Geometry check sheet. Reference: the model listing, model coordinates, mm. A direction names the side the tool comes from. Round coordinates to 2 decimals unless told otherwise and drop trailing zeros. Loops run counter-clockwise (first coordinate to the right, second up) from the corner with the lowest first, then second, coordinate; pieces in that order, holes last.
```python
from build123d import *

# Parameters (mm, degrees)
SKETCH_1_W          = 27.7
SKETCH_1_H          = 27.5
EXTRUDE_1_DEPTH     = 2
SKETCH_1_13_W       = 2
SKETCH_1_13_H       = 27.5
EXTRUDE_2_DEPTH     = 5
SKETCH_2_R          = 0.75
SKETCH_2_W          = 18
SKETCH_2_H          = 4.15
CUT_EXTRUDE_1_DEPTH = 22.196344024
SKETCH_2_3_W        = 25
SKETCH_2_3_H        = 19
CUT_EXTRUDE_2_DEPTH = 1
EXTRUDE_START       = 5
SKETCH_1_14_W       = 3
SKETCH_1_14_H       = 3
SKETCH_1_14_R       = 0.6
EXTRUDE_3_DEPTH     = 1.5


with BuildPart() as part:
    # 草图1 → 凸台-拉伸1 (new body)
    with BuildSketch(Plane.XY):
        Rectangle(SKETCH_1_W, SKETCH_1_H)
    extrude(amount=EXTRUDE_1_DEPTH)

    # 草图1<13> → 凸台-拉伸2 (add)
    with BuildSketch(Plane.XY):
        with Locations((-14.85, 0)):
            Rectangle(SKETCH_1_13_W, SKETCH_1_13_H)
        with Locations((14.85, 0)):
            Rectangle(SKETCH_1_13_W, SKETCH_1_13_H)
    extrude(amount=EXTRUDE_2_DEPTH)

    # 草图2 → 切除-拉伸1 (cut, through all)
    with BuildSketch(Plane.XY.offset(2)):
        with Locations((-11.7, 11.675)):
            Circle(SKETCH_2_R)
        with Locations((11.7, 11.675)):
            Circle(SKETCH_2_R)
        with Locations((-11.7, -11.675)):
            Circle(SKETCH_2_R)
        with Locations((11.7, -11.675)):
            Circle(SKETCH_2_R)
        with Locations((0, 11.675)):
            Rectangle(SKETCH_2_W, SKETCH_2_H)
    extrude(amount=-CUT_EXTRUDE_1_DEPTH, mode=Mode.SUBTRACT)

    # 草图2<3> → 切除-拉伸2 (cut)
    with BuildSketch(Plane.XY.offset(2)):
        with Locations((0, 0.1)):
            Rectangle(SKETCH_2_3_W, SKETCH_2_3_H)
    extrude(amount=-CUT_EXTRUDE_2_DEPTH, mode=Mode.SUBTRACT)

    # 草图1<14> → 凸台-拉伸3 (add)
    # profile 1 of 4: a face of its own
    with BuildSketch(Plane.XY.offset(EXTRUDE_START)):
        with Locations((-17.35, 12.25)):
            Rectangle(SKETCH_1_14_W, SKETCH_1_14_H)
        with Locations((-17.35, 12.25)):
            Circle(SKETCH_1_14_R, mode=Mode.SUBTRACT)
    # profile 2 of 4: a face of its own
    with BuildSketch(Plane.XY.offset(EXTRUDE_START)):
        with Locations((-17.35, -12.25)):
            Rectangle(SKETCH_1_14_W, SKETCH_1_14_H)
        with Locations((-17.35, -12.25)):
            Circle(SKETCH_1_14_R, mode=Mode.SUBTRACT)
    # profile 3 of 4: a face of its own
    with BuildSketch(Plane.XY.offset(EXTRUDE_START)):
        with Locations((17.35, -12.25)):
            Rectangle(SKETCH_1_14_W, SKETCH_1_14_H)
        with Locations((17.35, -12.25)):
            Circle(SKETCH_1_14_R, mode=Mode.SUBTRACT)
    # profile 4 of 4: a face of its own
    with BuildSketch(Plane.XY.offset(EXTRUDE_START)):
        with Locations((17.35, 12.25)):
            Rectangle(SKETCH_1_14_W, SKETCH_1_14_H)
        with Locations((17.35, 12.25)):
            Circle(SKETCH_1_14_R, mode=Mode.SUBTRACT)
    extrude(amount=-EXTRUDE_3_DEPTH)


solid = part.part
```
1) Sectioned sample at D-D, the plane y = -5.5. Record the cut outline in (x, z), then the cut area to 3 significant figures.
Report:
outline: (-15.85, 0) - (15.85, 0) - (15.85, 5) - (13.85, 5) - (13.85, 2) - (12.5, 2) - (12.5, 1) - (-12.5, 1) - (-12.5, 2) - (-13.85, 2) - (-13.85, 5) - (-15.85, 5) - close
area: 50.4 mm2
2) Sectioned sample at A-A, the plane z = 4.55. Record the cut outline in (x, y).
Report:
outline: (-18.85, -13.75) - (-13.85, -13.75) - (-13.85, 13.75) - (-18.85, 13.75) - (-18.85, 10.75) - (-15.85, 10.75) - (-15.85, -10.75) - (-18.85, -10.75) - close; (13.85, -13.75) - (18.85, -13.75) - (18.85, -10.75) - (15.85, -10.75) - (15.85, 10.75) - (18.85, 10.75) - (18.85, 13.75) - (13.85, 13.75) - close; hole circle Ø1.2 at (-17.35, -12.25); hole circle Ø1.2 at (-17.35, 12.25); hole circle Ø1.2 at (17.35, -12.25); hole circle Ø1.2 at (17.35, 12.25)
3) Scan lines: line 1 along Y through (x, z) = (-11.7, 1.3) (3 decimals); line 2 along Y through (x, z) = (-11.7, 0.8) (3 decimals); line 3 along X through (y, z) = (-7.75, 4.05). Record each from-to range of solid material in increasing order.
Report:
line 1: y = -13.75 to -12.425, -10.925 to -9.4, 9.6 to 10.925, 12.425 to 13.75
line 2: y = -13.75 to -12.425, -10.925 to 10.925, 12.425 to 13.75
line 3: x = -15.85 to -13.85, 13.85 to 15.85
4) Sectioned sample at B-B, the plane x = 11.7. Record the cut outline in (y, z) (3 decimals).
Report:
outline: (-13.75, 0) - (-12.425, 0) - (-12.425, 2) - (-13.75, 2) - close; (-10.925, 0) - (10.925, 0) - (10.925, 2) - (9.6, 2) - (9.6, 1) - (-9.4, 1) - (-9.4, 2) - (-10.925, 2) - close; (12.425, 0) - (13.75, 0) - (13.75, 2) - (12.425, 2) - close
5) Access from +Z, -Z, +X, -X, +Y, -Y to the whole of each face (thin tool, end or side, straight path). Record for faces 1 (the face through (17, -10.75, 4)), 2 (the face through (17, -13, 3.5)), 3 (the face through (13.85, 0, 3)), 4 (the face through (-0.1, 9.6, 0.5)), 5 (the face through (12.5, 0, 1.5)).
Report:
face 1: +Z, -Z, +X
face 2: -Z, +X, +Y, -Y
face 3: +Z, +Y, -Y
face 4: +Z, -Z, +Y
face 5: +Z
6) Gauge pin test, flat ends, axial feed: pin 1 (0.9 mm diameter, centred on x = 17, y = 13, fed in from -Z); pin 2 (1.2 mm diameter, centred on x = -11.7, y = -11.675, fed in from -Z); pin 3 (3 mm diameter, centred on y = 6.5, z = 3, fed in from +X); pin 4 (1.7 mm diameter, centred on x = -11.7, y = 11.675, fed in from +Z). Record the tip position at first contact, or that the pin passes through.
Report:
pin 1: stops at z = 3.5
pin 2: passes through
pin 3: stops at x = 15.85
pin 4: stops at z = 2
7) Mould release check, pull along X, two halves, no side actions. Record for faces 6 (the face through (-18.85, -12, 4)), 7 (the face through (17, 10.75, 4)), 8 (the face through (0, -10, 2)): +X half, -X half, draft (parallel to the pull), parting line (faces both ways), or undercut.
Report:
face 6: -X half
face 7: draft
face 8: undercut
8) Sectioned sample at C-C, the plane x = 17.35. Record the cut outline in (y, z), then the cut area to 3 significant figures.
Report:
outline: (-13.75, 3.5) - (-12.85, 3.5) - (-12.85, 5) - (-13.75, 5) - close; (-11.65, 3.5) - (-10.75, 3.5) - (-10.75, 5) - (-11.65, 5) - close; (10.75, 3.5) - (11.65, 3.5) - (11.65, 5) - (10.75, 5) - close; (12.85, 3.5) - (13.75, 3.5) - (13.75, 5) - (12.85, 5) - close
area: 5.40 mm2
